Design review of the part built by this model. Coordinates are the model's own, in mm. Give positions to 0.01 mm unless a question says otherwise; leave off trailing zeros. Write each loop counter-clockwise with the first axis right and the second up, starting at its lowest first coordinate (ties: lowest second). Pieces come first, ordered by that corner, then holes. Notation, with made-up numbers: (70, 75) -> (99, 75) arc R22 ccw to (99, 81) -> close; hole circle Ø7 at (-7, -4.5). An arc over 180 degrees is marked (long way). Answer as a JSON object with one key per item and string values.
Autodesk Inventor part; units mm, degrees
ref_plane "YZ Plane" through (0, 0, 0) normal (1, 0, 0) x (0, 1, 0)
ref_plane "XZ Plane" through (0, 0, 0) normal (0, 1, 0) x (-1, 0, 0)
ref_plane "XY Plane" through (0, 0, 0) normal (0, 0, 1) x (1, 0, 0)
sketch "Sketch1" plane through (0, 0, 0) normal (0, 1, 0) x (-1, 0, 0)
  line L0 (20, 45) -> (-20, 45)
  line L1 (-20, 45) -> (-20, -45)
  line L2 (-20, -45) -> (20, -45)
  line L3 (20, -45) -> (20, 45)
  line L4 (20, 45) -> (-20, -45) construction
  line L5 (-20, 45) -> (20, -45) construction
  circle A0 centre (0, 0) radius 15.5
  line L6 (0, 0) -> (0, -19.5)
  line L7 (0, -19.5) -> (0, 19.5)
  circle A1 centre (0, 19.5) radius 1.5
  circle A2 centre (0, -19.5) radius 1.5
  line L8 (15, 40) -> (-15, 40)
  line L9 (-15, 40) -> (-15, -40)
  line L10 (-15, -40) -> (15, -40)
  line L11 (15, -40) -> (15, 40)
  line L12 (15, 40) -> (-15, -40) construction
  line L13 (-15, 40) -> (15, -40) construction
  circle A3 centre (15, 40) radius 2
  circle A4 centre (15, -40) radius 2
  circle A5 centre (-15, -40) radius 2
  circle A6 centre (-15, 40) radius 2
  dimension "d0" = 40
  dimension "d1" = 90
  dimension "d2" = 31
  dimension "d3" = 19.5
  dimension "d4" = 39
  dimension "d5" = 3
  dimension "d6" = 3
  dimension "d9" = 30
  dimension "d10" = 80
  dimension "d11" = 4
  dimension "d12" = 4
  dimension "d13" = 4
  dimension "d14" = 4
extrude "Extrusion1" add sketch "Sketch1" along normal blind 4.5 contours L3 L2 L1 L0 | A0 L9 A6 L8 A3 L11 | L11 A4 L10 A5 L9 A0
properties part number "caster_holder"
(1) For line 1 along Z through (x, y) = (0, 2.1); line 2 along X through (y, z) = (1.2, -40); line 3 along Z through (x, y) = (-16, 2.35), list the stretches that pass through material, from the lowest coordinate up.
Here are the results:
{"line 1": "z = -45 to -21, -18 to -15.5, 15.5 to 18, 21 to 45", "line 2": "x = -20 to -17, -13 to 13, 17 to 20", "line 3": "z = -45 to -41.73, -38.27 to 38.27, 41.73 to 45"}
(2) The part is to be moulded in two halves that separate along X. For faces 1 (the flat face through (-20, 2, -1)), 2 (the cylindrical face through (-15, 2, 42)), 3 (the flat face through (0, 2, 45)), say which applies: +X half, -X half, draft (parallel to the pull), parting line (faces both ways), or undercut.
Here are the results:
{"face 1": "-X half", "face 2": "undercut", "face 3": "draft"}
(3) We need section C-C, the plane y = 1.7. State the section outline as (x, z) points, then the cut area to 3 significant figures.
Here are the results:
{"outline": "(-20, -45) -> (20, -45) -> (20, 45) -> (-20, 45) -> close; hole circle Ø4 at (-15, -40); hole circle Ø4 at (-15, 40); hole circle Ø31 at (0, 0); hole circle Ø3 at (0, -19.5); hole circle Ø3 at (0, 19.5); hole circle Ø4 at (15, -40); hole circle Ø4 at (15, 40)", "area": "2,780 mm²"}
(4) We need section A-A, the plane x = 0. State the section outline as (y, z) points.
Here are the results:
{"outline": "(0, -45) -> (4.5, -45) -> (4.5, -21) -> (0, -21) -> close; (0, -18) -> (4.5, -18) -> (4.5, -15.5) -> (0, -15.5) -> close; (0, 15.5) -> (4.5, 15.5) -> (4.5, 18) -> (0, 18) -> close; (0, 21) -> (4.5, 21) -> (4.5, 45) -> (0, 45) -> close"}
(5) We need section B-B, the plane z = 19.5. State the section outline as (x, y) points, then the cut area to 4 significant figures.
Here are the results:
{"outline": "(-20, 0) -> (-1.5, 0) -> (-1.5, 4.5) -> (-20, 4.5) -> close; (1.5, 0) -> (20, 0) -> (20, 4.5) -> (1.5, 4.5) -> close", "area": "166.5 mm²"}
(6) We need section D-D, the plane z = -40. State the section outline as (x, y) points, then the cut area to 3 significant figures.
Here are the results:
{"outline": "(-20, 0) -> (-17, 0) -> (-17, 4.5) -> (-20, 4.5) -> close; (-13, 0) -> (13, 0) -> (13, 4.5) -> (-13, 4.5) -> close; (17, 0) -> (20, 0) -> (20, 4.5) -> (17, 4.5) -> close", "area": "144 mm²"}
